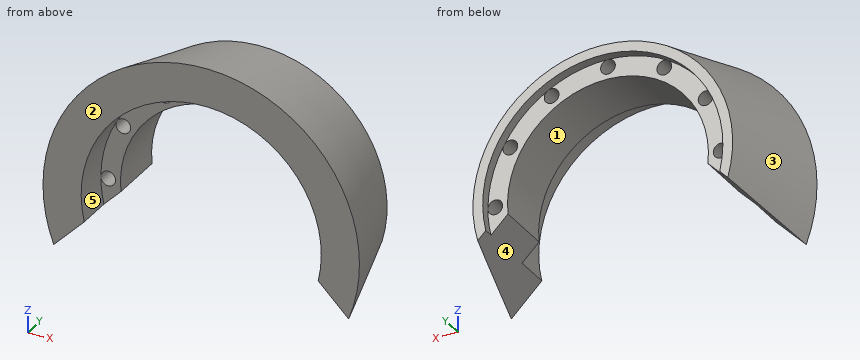
```python
from build123d import *

# Parameters (mm, degrees)
SKETCH2_R               = 4.7625
CUT_EXTRUDE1_DEPTH      = 63.23
CIRPATTERN1_COUNT       = 12
CUT_EXTRUDE2_DEPTH      = 26.4
CUT_EXTRUDE2_DEPTH_BACK = 44.18


with BuildPart() as part:
    # Sketch1 → Revolve1 (revolve)
    with BuildSketch(Plane(origin=(0, 0, 0), x_dir=(0, 0, -1), z_dir=(1, 0, 0))):
        Polygon((65.0875, -19.05), (65.0875, 19.05), (77.7875, 19.05), (77.7875, 25.4), (84.1375, 25.4), (102.513455617, -43.18), (77.7875, -43.18), (77.7875, -25.4), (77.7875, -19.05), align=None)
    revolve(axis=Axis((0, -44.45, 0), (0, 1, 0)))

    # Sketch2 → Cut-Extrude1 (cut, through all)
    with BuildSketch(Plane(origin=(0, 19.05, 0), x_dir=(1, 0, 0), z_dir=(0, 1, 0))):
        with Locations((0, -73.025)):
            Circle(SKETCH2_R)
    cut_extrude1 = extrude(amount=-CUT_EXTRUDE1_DEPTH, mode=Mode.SUBTRACT)

    # CirPattern1: Cut-Extrude1 ×12 about axis
    cirpattern1_axis = Axis((0, 0, 0), (0, 1, 0))
    for i in range(1, CIRPATTERN1_COUNT):
        add(cut_extrude1.rotate(cirpattern1_axis, i * 360 / CIRPATTERN1_COUNT), mode=Mode.SUBTRACT)

    # Sketch3 → Cut-Extrude2 (cut, two sides)
    with BuildSketch(Plane(origin=(0, 0, 0), x_dir=(1, 0, 0), z_dir=(0, 1, 0))) as cut_extrude2_sk:
        with BuildLine():
            Line((0, -58.371664787), (95.538612884, 37.166948097))
            ThreePointArc((95.538612884, 37.166948097), (0, 102.513455617), (-95.538612884, 37.166948097))
            Line((-95.538612884, 37.166948097), (0, -58.371664787))
        make_face()
    extrude(amount=CUT_EXTRUDE2_DEPTH, mode=Mode.SUBTRACT)
    extrude(cut_extrude2_sk.sketch, amount=-CUT_EXTRUDE2_DEPTH_BACK, mode=Mode.SUBTRACT)


solid = part.part
```
Design review of the part built by this model. Coordinates are the model's own, in mm. Face numbers are marked on the shaded views. A direction names the side the tool comes from. Round coordinates to 2 decimals unless told otherwise and drop trailing zeros. Order: outer loops, then holes, each group sorted by start corner. A loop starts at its lowest first (then second) coordinate and runs counter-clockwise, first axis right, second up. Notation, with made-up numbers: (-10.75, 84.5) - (7.25, 84.5) arc R21 ccw to (7.25, 118.5) - close; hole circle Ø11 at (82, -2). An arc over 180 degrees is marked (long way). One line per question, with ' | ' between items.
Item 1: Draft analysis for pull direction X (two halves, no side actions). For the marked faces 1, 2 and 3, state which applies: +X half, -X half, draft (parallel to the pull), parting line (faces both ways), or undercut.
Checks:
face 1: undercut | face 2: draft | face 3: parting line
Item 2: Wall thickness on line 1 (Y direction, x = -45, z = 54.5); line 2 (X direction, y = 20.5, z = 42); line 3 (X direction, y = -13.5, z = 73.5): over which ranges is each line inside the solid? List them lowest first. Write a range as [from, to].
Checks:
line 1: [-19.05, 19.05] | line 2: [-74.42, -65.47], [65.47, 74.42] | line 3: [-59.49, -4.74], [4.74, 59.49]
Item 3: Machinability: for the marked faces 4 and 5, which of the approach directions +Z, -Z, +X, -X, +Y, -Y give a long, thin tool a straight path to every point of the face, cutting with its end or side? Answer none if there is none.
Checks:
face 4: -Z, +Y, -Y | face 5: -Y
Item 4: Take a section at B-B, the plane y = -25. Write out the cut boundary in (x, z) (1 decimal), then the cut area to 3 significant figures.
Checks:
outline: (-91.8, -33.4) - (-75.8, -17.4) arc R77.8 cw (long way) to (75.8, -17.4) - (91.8, -33.4) arc R97.6 ccw (long way) to start | area: 6,500 mm²
Item 5: Take a section at A-A, the plane y = -10.5. Write out the cut boundary in (x, z) (1 decimal), then the cut area to 3 significant figures.
Checks:
outline: (-88.7, -30.3) - (-64.8, -6.4) arc R65.1 cw (long way) to (64.8, -6.4) - (88.7, -30.3) arc R93.8 ccw (long way) to start; hole circle Ø9.5 at (-73, 0); hole circle Ø9.5 at (-63.2, 36.5); hole circle Ø9.5 at (-36.5, 63.2); hole circle Ø9.5 at (0, 73); hole circle Ø9.5 at (36.5, 63.2); hole circle Ø9.5 at (63.2, 36.5); hole circle Ø9.5 at (73, 0) | area: 7,740 mm²
Item 6: For P1, Ø7.5, axis at x = 0, z = 73.025, coming from the -Y side; P2, Ø4, axis at x = 25, y = 11, coming from the +Z side; P3, Ø5, axis at y = 3.5, z = 32, coming from the -X side; P4, Ø3, axis at y = -11, z = 48.5, coming from the -X side, all flat-tipped, find the tip position at first contact; note any pin that passes through.
Checks:
P1: through | P2: z = 85.17 | P3: x = -85.29 | P4: x = -81.4
